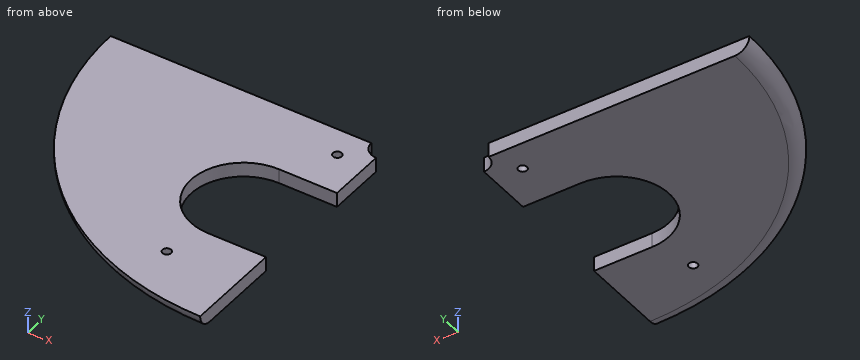
```python
from build123d import *

# Parameters (mm, degrees)
SKETCH_1_R          = 1.5
EXTRUDE_1_DEPTH     = 5
CUT_EXTRUDE_1_DEPTH = 135.443296597
FILLET_2_R          = 5


with BuildPart() as part:
    # 草圖1 → 填料-伸長1 (new body)
    with BuildSketch(Plane.XY):
        with BuildLine():
            Line((-5, 0), (-95, 0))
            ThreePointArc((-95, 0), (-67.175144213, -67.175144213), (0, -95))
            Line((0, -95), (0, -5))
            ThreePointArc((0, -5), (-3.535533906, -3.535533906), (-5, 0))
        make_face()
        with Locations((-10, -10)):
            Circle(SKETCH_1_R, mode=Mode.SUBTRACT)
        with Locations((-25, -75)):
            Circle(SKETCH_1_R, mode=Mode.SUBTRACT)
    extrude(amount=EXTRUDE_1_DEPTH)

    # 草圖2 → 除料-伸長1 (cut, through all)
    with BuildSketch(Plane(origin=(0, 0, 0), x_dir=(-1, 0, 0), z_dir=(0, 0, -1))):
        with BuildLine():
            Line((0, -25), (0, -61.312071511))
            Line((0, -61.312071511), (20, -61.312071511))
            ThreePointArc((20, -61.312071511), (38.156035755, -43.156035755), (20, -25))
            Line((20, -25), (0, -25))
        make_face()
    extrude(amount=-CUT_EXTRUDE_1_DEPTH, mode=Mode.SUBTRACT)

    # 圓角2
    fillet_2_edges = [part.edges().sort_by_distance(p)[0] for p in [
        (-67.175144213, -67.175144213, 0),
    ]]
    fillet(fillet_2_edges, radius=FILLET_2_R - 0.0001)  # a hair under: the kernel refuses the full size


solid = part.part
```
Verification items for the finished model (mm, model axes). Coordinates: 2 decimals unless noted, no trailing zeros. Loops run counter-clockwise (first coordinate to the right, second up) from the corner with the lowest first, then second, coordinate; pieces in that order, holes last. Notation, with made-up numbers: (10.25, 19.5) -> (21.25, 19.5) arc R20 ccw to (21.25, 44.5) -> close; hole circle Ø7 at (67.25, 74.5). An arc over 180 degrees is marked (long way). Answer in a Markdown table with one row per item. Add a question column.
1. Material ranges on probe 1 along Y at (x, z) = (-10, 1.7); probe 2 along Y at (x, z) = (-25, 1.85); probe 3 along X at (y, z) = (-75, 1.85), recorded low to high. Write a range as [from, to].
2. Depth check by flat-ended pin: P1, Ø1, axis at x = -37, y = -46.5, coming from the -Z side; P2, Ø1.5, axis at x = -12, z = 3, coming from the -Y side; P3, Ø3, axis at y = -27.5, z = 2.5, coming from the -X side. Enter the tip coordinate at first touch or a pass-through.
3. Section check B-B, the plane x = -25. Give the number of separate pieces and of enclosed holes in the cut face, then the cut area to 3 significant figures.
4. Section check A-A, the plane z = 1.6. Enter the section's corners in (x, y), then the cut area to 3 significant figures.
Derived:
| question | item | result |
|---|---|---|
| 1 | probe 1 | y = [-93.22, -61.31], [-25, -11.5], [-8.5, 0] |
| 1 | probe 2 | y = [-90.49, -76.5], [-73.5, -60.61], [-25.7, 0] |
| 1 | probe 3 | x = [-56.47, -26.5], [-23.5, 0] |
| 2 | P1 | passes through |
| 2 | P2 | stops at y = -94.1 |
| 2 | P3 | stops at x = -91.03 |
| 3 | separate pieces | 3 |
| 3 | enclosed holes | 0 |
| 3 | area | 263 mm² |
| 4 | outline | (-93.67, 0) arc R93.67 ccw to (0, -93.67) -> (0, -61.31) -> (-20, -61.31) arc R18.16 cw to (-20, -25) -> (0, -25) -> (0, -5) arc R5 cw to (-5, 0) -> close; hole circle Ø3 at (-25, -75); hole circle Ø3 at (-10, -10) |
| 4 | area | 5,610 mm² |
